Work out the finished part from the listing and answer in its coordinate system (mm). A direction names the side the tool comes from. Round coordinates to 2 decimals unless told otherwise and drop trailing zeros. Write each loop counter-clockwise with the first axis right and the second up, starting at its lowest first coordinate (ties: lowest second). Pieces come first, ordered by that corner, then holes.
1. A tool of negligible diameter and unlimited length cuts with its end or side. For faces 4 (the face through (222.25, -38, 4)), 5 (the face through (113, -76.2, 4)), 6 (the face through (139, -38, 5.08)), from which of +Z, -Z, +X, -X, +Y, -Y can it reach the whole face along a straight path? Write none if from no direction.
2. Find section A-A (x = 44.45). Write down the section's boundary in (y, z) (3 decimals).
3. Straight lines are drawn through the part: probe 1 along Y at (x, z) = (44.45, 2) (3 decimals); probe 2 along Y at (x, z) = (204, 6.25); probe 3 along X at (y, z) = (-7, 4). For each, find the intervals that lie inside material, in ascending order.
4. A flat-ended cylindrical pin translates along its axis: pin 1 Ø3 at (x, z) = (215.9, 4.191) entering from +Y (3 decimals). Find the tip coordinate at first contact, or state that the pin passes through.
5. Find section B-B (x = 94). Write down the section's boundary in (y, z).
6. Determine the mould class of faces 1 (the face through (113, 0, 4)), 2 (the face through (228.6, -38, 4)), 3 (the face through (43.76, -34.85, 4.25)) for opening direction X: pulls with the +X half, pulls with the -X half, needs draft (parallel to the pull), parting line crosses it, or undercut.
```python
from build123d import *

# Parameters (mm, degrees)
F0_W     = 228.6
F0_H     = 8.382
F1_DEPTH = 76.2
F2_R     = 1.5875
F3_DEPTH = 76.201
F4_W     = 25.4
F4_H     = 25.4
F4_R     = 3.175
F5_DEPTH = 8.383
F6_W     = 114.3
F6_H     = 12.7
F7_DEPTH = 5.08


with BuildPart() as f1:
    # F0 (on Front) → F1 (new body)
    with BuildSketch(Plane.XZ):
        with Locations((114.3, 4.191)):
            Rectangle(F0_W, F0_H)
    extrude(amount=F1_DEPTH)

    # F2 (on face) → F3 (cut, through all)
    with BuildSketch(Plane.XZ.offset(76.2)):
        with Locations((12.7, 4.191)):
            Circle(F2_R)
        with Locations((215.9, 4.191)):
            Circle(F2_R)
    extrude(amount=-F3_DEPTH, mode=Mode.SUBTRACT)

    # F4 (on face) → F5 (cut, through all)
    with BuildSketch(Plane.XY.offset(8.382)):
        with Locations((209.55, -38.1)):
            Rectangle(F4_W, F4_H)
        with Locations((44.45, -31.75)):
            Circle(F4_R)
        with Locations((44.45, -44.45)):
            Circle(F4_R)
    extrude(amount=-F5_DEPTH, mode=Mode.SUBTRACT)

    # F6 (on face) → F7 (cut)
    with BuildSketch(Plane(origin=(0, 0, 0), x_dir=(1, 0, 0), z_dir=(0, 0, -1))):
        with Locations((139.7, 38.1)):
            Rectangle(F6_W, F6_H)
    extrude(amount=-F7_DEPTH, mode=Mode.SUBTRACT)


solid = f1.part
```
Worked answers:
1. face 4: +Z, -Z
1. face 5: +Z, -Z, +X, -X, -Y
1. face 6: -Z
2. outline: (-76.2, 0) - (-47.625, 0) - (-47.625, 8.382) - (-76.2, 8.382) - close; (-41.275, 0) - (-34.925, 0) - (-34.925, 8.382) - (-41.275, 8.382) - close; (-28.575, 0) - (0, 0) - (0, 8.382) - (-28.575, 8.382) - close
3. probe 1: y = -76.2 to -47.625, -41.275 to -34.925, -28.575 to 0
3. probe 2: y = -76.2 to -50.8, -25.4 to 0
3. probe 3: x = 0 to 11.12, 14.28 to 214.32, 217.48 to 228.6
4. pin 1: passes through
5. outline: (-76.2, 0) - (-44.45, 0) - (-44.45, 5.08) - (-31.75, 5.08) - (-31.75, 0) - (0, 0) - (0, 8.38) - (-76.2, 8.38) - close
6. face 1: needs draft
6. face 2: pulls with the +X half
6. face 3: undercut
